Work out the finished part from the listing and answer in its coordinate system (mm). Face numbers are marked on the shaded views. A direction names the side the tool comes from. Coordinates: 2 decimals unless noted, no trailing zeros. Order: outer loops, then holes, each group sorted by start corner. A loop starts at its lowest first (then second) coordinate and runs counter-clockwise, first axis right, second up. Notation, with made-up numbers: M -8.75,75 L 40.25,75 A13 cw 40.25,87 Z; hole C 88.25,18 d2. An arc over 180 degrees is marked long. Write item = value, one per line. Start each with the question number.
Q1. A tool of negligible diameter and unlimited length cuts with its end or side. For the marked faces 1 and 2, from which of +Z, -Z, +X, -X, +Y, -Y can it reach the whole face along a straight path? Write none if from no direction.
Q2. Each of these flat-tipped pins is pushed along its axis until it touches: P1, Ø3, axis at y = -4.5, z = 2.5, coming from the +X side; P2, Ø4, axis at x = -20, y = 0, coming from the -Z side; P3, Ø4, axis at x = 20.5, y = 0.5, coming from the +Z side. Where does it stop, or does it pass through?
Q3. Find section A-A on x = 0. Give the number of separate pieces and of enclosed holes in the cut face, and give its area (3 significant figures).
Q4. Straight lines are drawn through the part: line 1 along Y through (x, z) = (1, 1.25); line 2 along Y through (x, z) = (20, 1.8); line 3 along Z through (x, y) = (-16.5, 11). For each, find the intervals that lie inside material, in ascending order.
Q5. Determine the mould class of the marked faces 3 and 4 for opening direction X: released by +X, released by -X, zero draft, split by the parting line, or undercut.
Q6. Find section C-C on z = 10. Give the vertices of the cut face in (x, y).
```python
from build123d import *

# Parameters (mm, degrees)
TORUS_R              = 1.5
ARRAY003_Z_COUNT     = 2
ARRAY003_Z_PITCH     = 6
CYLINDER004001_R     = 4.5
CYLINDER004001_DEPTH = 0.2
ARRAY002_COUNT       = 2
CYLINDER004_R        = 4.5
CYLINDER004_DEPTH    = 10
ARRAY001_COUNT       = 2
CYLINDER001_R        = 1.8
CYLINDER001_DEPTH    = 10
ARRAY_COUNT          = 8
CYLINDER003_R        = 4.5
CYLINDER003_DEPTH    = 14
CYLINDER002_R        = 5.5
CYLINDER002_DEPTH    = 10
CYLINDER_R           = 30
CYLINDER_DEPTH       = 15


with BuildPart() as array_torus:
    # Torus → Torus (revolve)
    with BuildSketch(Plane(origin=(0, 0, -1.5), x_dir=(1, 0, 0), z_dir=(0, -1, 0))):
        with Locations((30, 0)):
            Circle(TORUS_R)
    revolve(axis=Axis((0, 0, -1.5), (0, 0, 1)))

    # Array003 Z: Array_torus ×2


with BuildPart() as array_torus_1:
    add(array_torus.part)
    with Locations(*[(0, 0, i * ARRAY003_Z_PITCH) for i in range(1, ARRAY003_Z_COUNT)]):
        add(array_torus.part)


with BuildPart() as array_torus_2:
    # Array003 placement: moved
    add(array_torus_1.part.moved(Location((0, 0, 6))))


with BuildPart() as cap_cover_thin:
    # Cylinder004001 → Cylinder004001 (new body)
    with BuildSketch(Plane(origin=(20, 0, 0.8), x_dir=(1, 0, 0), z_dir=(0, 0, 1))):
        Circle(CYLINDER004001_R)
    extrude(amount=CYLINDER004001_DEPTH)

    # Array002: cap-cover-thin ×2 about axis
    array002_axis = Axis((0, 0, 0), (0, 0, 1))


with BuildPart() as cap_cover_thin_1:
    add(cap_cover_thin.part)
    for i in range(1, ARRAY002_COUNT):
        add(cap_cover_thin.part.rotate(array002_axis, i * 360 / ARRAY002_COUNT))


with BuildPart() as cap_cover_thin_2:
    # Array002 placement: moved
    add(cap_cover_thin_1.part.moved(Location((0, 0, 2))))


with BuildPart() as cutout_for_screws_cap:
    # Cylinder004 → Cylinder004 (new body)
    with BuildSketch(Plane(origin=(20, 0, -9), x_dir=(1, 0, 0), z_dir=(0, 0, 1))):
        Circle(CYLINDER004_R)
    extrude(amount=CYLINDER004_DEPTH)

    # Array001: Cutout-for-screws-cap ×2 about axis
    array001_axis = Axis((0, 0, 0), (0, 0, 1))


with BuildPart() as cutout_for_screws_cap_1:
    add(cutout_for_screws_cap.part)
    for i in range(1, ARRAY001_COUNT):
        add(cutout_for_screws_cap.part.rotate(array001_axis, i * 360 / ARRAY001_COUNT))


with BuildPart() as cutout_for_screws_cap_2:
    # Array001 placement: moved
    add(cutout_for_screws_cap_1.part.moved(Location((0, 0, 2))))


with BuildPart() as cylinders_array_drills:
    # Cylinder001 → Cylinder001 (new body)
    with BuildSketch(Plane(origin=(20, 0, -2), x_dir=(1, 0, 0), z_dir=(0, 0, 1))):
        Circle(CYLINDER001_R)
    extrude(amount=CYLINDER001_DEPTH)

    # Array: Cylinders-array-drills ×8 about axis
    array_axis = Axis((0, 0, 0), (0, 0, 1))


with BuildPart() as cylinders_array_drills_1:
    add(cylinders_array_drills.part)
    for i in range(1, ARRAY_COUNT):
        add(cylinders_array_drills.part.rotate(array_axis, i * 360 / ARRAY_COUNT))


with BuildPart() as cylinder_inner_shaft:
    # Cylinder003 → Cylinder003 (new body)
    with BuildSketch(Plane.XY.offset(-1)):
        Circle(CYLINDER003_R)
    extrude(amount=CYLINDER003_DEPTH)


with BuildPart() as inner_cutout_4_5mm:
    # Cylinder002 → Cylinder002 (new body)
    with BuildSketch(Plane.XY.offset(1.3)):
        Circle(CYLINDER002_R)
    extrude(amount=CYLINDER002_DEPTH)


with BuildPart() as conic_cutout:
    # Cone → Cone (revolve)
    with BuildSketch(Plane(origin=(0, 0, 15), x_dir=(-1, 0, 0), z_dir=(0, -1, 0))):
        Polygon((0, 0), (28, 0), (25, 10), (0, 10), align=None)
    revolve(axis=Axis((0, 0, 15), (0, 0, -1)))


with BuildPart() as wheel_rear:
    # Cylinder → Cylinder (new body)
    with BuildSketch(Plane.XY):
        Circle(CYLINDER_R)
    extrude(amount=CYLINDER_DEPTH)

    # Cut: cut conic-cutout
    add(conic_cutout.part, mode=Mode.SUBTRACT)

    # Cut001: cut inner-cutout-4.5mm
    add(inner_cutout_4_5mm.part, mode=Mode.SUBTRACT)

    # Cut002: cut cylinder-inner-shaft
    add(cylinder_inner_shaft.part, mode=Mode.SUBTRACT)

    # Cut003: cut Cylinders-array-drills
    add(cylinders_array_drills_1.part, mode=Mode.SUBTRACT)

    # Cut004: cut Cutout-for-screws-cap
    add(cutout_for_screws_cap_2.part, mode=Mode.SUBTRACT)

    # Fusion: union cap-cover-thin
    add(cap_cover_thin_2.part)

    # Cut005: cut Array_torus
    add(array_torus_2.part, mode=Mode.SUBTRACT)


solid = wheel_rear.part
```
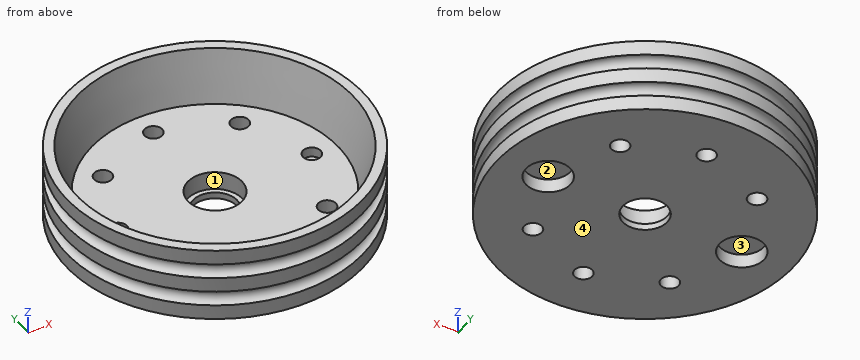
Findings below:
q1.face_1 = +Z
q1.face_2 = -Z
q2.P1 = 29.85
q2.P2 = 2.8
q2.P3 = 5
q3.separate_pieces = 4
q3.enclosed_holes = 0
q3.area = 267 mm^2
q4.line_1 = -29.98 to -21.5, -18.5 to -4.39, 4.39 to 18.5, 21.5 to 29.98
q4.line_2 = -22.36 to -4.5, 4.5 to 22.36
q4.line_3 = 0 to 5
q5.face_3 = undercut
q5.face_4 = zero draft
q6.outline = C 0,0 d57.17; hole C 0,0 d53
